Verification items for the finished model (mm, model axes). Coordinates: 2 decimals unless noted, no trailing zeros. Order: outer loops, then holes, each group sorted by start corner. A loop starts at its lowest first (then second) coordinate and runs counter-clockwise, first axis right, second up.
Q1. Cross-section at B-B, the plane z = 737. Record the boundary of the cut face in (x, y).
Q2. Depth check by flat-ended pin: P1, Ø12, axis at y = -8.5, z = 2046, coming from the +X side; P2, Ø1, axis at y = 5.5, z = 1956.5, coming from the +X side; P3, Ø8, axis at x = -9, z = 1829.5, coming from the +Y side. Enter the tip coordinate at first touch or a pass-through.
Q3. Cross-section at A-A, the plane x = 0. Record the boundary of the cut face in (y, z), and give its area (3 significant figures).
Q4. Thickness scan on line 1 (Z direction, x = 9.5, y = -1.25); line 2 (Z direction, x = 9.75, y = 0); line 3 (Y direction, x = -1.75, z = 1896.5). Record the ranges inside material, lowest first.
from build123d import *

# Parameters (mm, degrees)
CROQUIS1_R                   = 12.5
CROQUIS1_R_2                 = 9.5
SALIENTE_EXTRUIR1_DEPTH      = 2380
SALIENTE_EXTRUIR1_DEPTH_BACK = 3
CROQUIS2_R                   = 3.43
CORTAR_EXTRUIR1_DEPTH        = 13.5
CORTAR_EXTRUIR1_DEPTH_BACK   = 13.5
CROQUIS3_R                   = 3.43
CORTAR_EXTRUIR2_DEPTH        = 13.5000001
CORTAR_EXTRUIR2_DEPTH_BACK   = 13.5000001


with BuildPart() as part:
    # Croquis1 → Saliente-Extruir1 (new body, two sides)
    with BuildSketch(Plane.XY) as saliente_extruir1_sk:
        Circle(CROQUIS1_R)
        Circle(CROQUIS1_R_2, mode=Mode.SUBTRACT)
    extrude(amount=SALIENTE_EXTRUIR1_DEPTH)
    extrude(saliente_extruir1_sk.sketch, amount=-SALIENTE_EXTRUIR1_DEPTH_BACK)

    # Croquis2 → Cortar-Extruir1 (cut, two sides)
    with BuildSketch(Plane(origin=(0, 0, 0), x_dir=(0, 0, -1), z_dir=(1, 0, 0))) as cortar_extruir1_sk:
        with Locations((-21, 0)):
            Circle(CROQUIS2_R)
    extrude(amount=CORTAR_EXTRUIR1_DEPTH, mode=Mode.SUBTRACT)
    extrude(cortar_extruir1_sk.sketch, amount=-CORTAR_EXTRUIR1_DEPTH_BACK, mode=Mode.SUBTRACT)

    # Croquis3 → Cortar-Extruir2 (cut, two sides)
    with BuildSketch(Plane(origin=(0, 0, 0), x_dir=(0, 0, -1), z_dir=(1, 0, 0))) as cortar_extruir2_sk:
        with Locations((-2356, 0)):
            Circle(CROQUIS3_R)
    extrude(amount=CORTAR_EXTRUIR2_DEPTH, mode=Mode.SUBTRACT)
    extrude(cortar_extruir2_sk.sketch, amount=-CORTAR_EXTRUIR2_DEPTH_BACK, mode=Mode.SUBTRACT)


solid = part.part
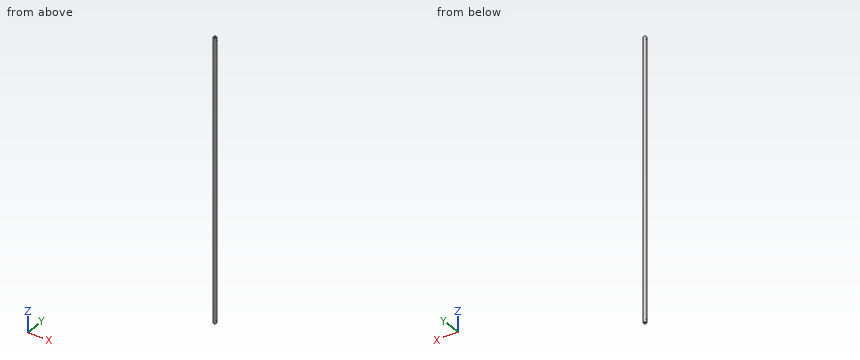
Check values:
1. outline: circle Ø25 at (0, 0); hole circle Ø19 at (0, 0)
2. P1: stops at x = 12.25
2. P2: stops at x = 11.46
2. P3: stops at y = 11.46
3. outline: (-12.5, -3) - (-9.5, -3) - (-9.5, 2380) - (-12.5, 2380) - close; (9.5, -3) - (12.5, -3) - (12.5, 2380) - (9.5, 2380) - close
3. area: 14,300 mm2
4. line 1: z = -3 to 17.81, 24.19 to 2352.81, 2359.19 to 2380
4. line 2: z = -3 to 17.57, 24.43 to 2352.57, 2359.43 to 2380
4. line 3: y = -12.38 to -9.34, 9.34 to 12.38
